from build123d import *

# Parameters (mm, degrees)
SKETCH2_R           = 45
BOSS_EXTRUDE3_DEPTH = 56
SKETCH4_W           = 90
SKETCH4_H           = 170
BOSS_EXTRUDE4_DEPTH = 30
SKETCH6_R           = 15
BOSS_EXTRUDE5_DEPTH = 170
SKETCH11_W          = 132.381260595
SKETCH11_H          = 110
CUT_EXTRUDE3_DEPTH  = 130


with BuildPart() as part:
    # Sketch2 → Boss-Extrude3 (new body)
    with BuildSketch(Plane.XY):
        Circle(SKETCH2_R)
        with BuildLine():
            Line((-4.5, 29.491665255), (4.5, 29.491665255))
            Line((4.5, 29.491665255), (4.5, 24.591665255))
            ThreePointArc((4.5, 24.591665255), (0, -25), (-4.5, 24.591665255))
            Line((-4.5, 24.591665255), (-4.5, 29.491665255))
        make_face(mode=Mode.SUBTRACT)
    extrude(amount=-BOSS_EXTRUDE3_DEPTH)

    # Sketch4 → Boss-Extrude4 (add)
    with BuildSketch(Plane(origin=(0, 0, -56), x_dir=(-1, 0, 0), z_dir=(0, 0, -1))):
        Rectangle(SKETCH4_W, SKETCH4_H)
    extrude(amount=BOSS_EXTRUDE4_DEPTH)

    # Sketch6 → Boss-Extrude5 (add)
    with BuildSketch(Plane(origin=(0, 85, 0), x_dir=(1, 0, 0), z_dir=(0, 1, 0))):
        with BuildLine():
            Line((45, 86), (38, 130))
            ThreePointArc((38, 130), (0, 168), (-38, 130))
            Line((-38, 130), (-45, 86))
            Line((-45, 86), (45, 86))
        make_face()
        with Locations(Location((0, 130, 0), (0, 0, 270))):
            Circle(SKETCH6_R, mode=Mode.SUBTRACT)
    extrude(amount=-BOSS_EXTRUDE5_DEPTH)

    # Sketch11 → Cut-Extrude3 (cut, symmetric)
    with BuildSketch(Plane(origin=(0, 0, 0), x_dir=(0, 0, -1), z_dir=(1, 0, 0))):
        with Locations((152.190630298, 0)):
            Rectangle(SKETCH11_W, SKETCH11_H)
    extrude(amount=CUT_EXTRUDE3_DEPTH, both=True, mode=Mode.SUBTRACT)


solid = part.part
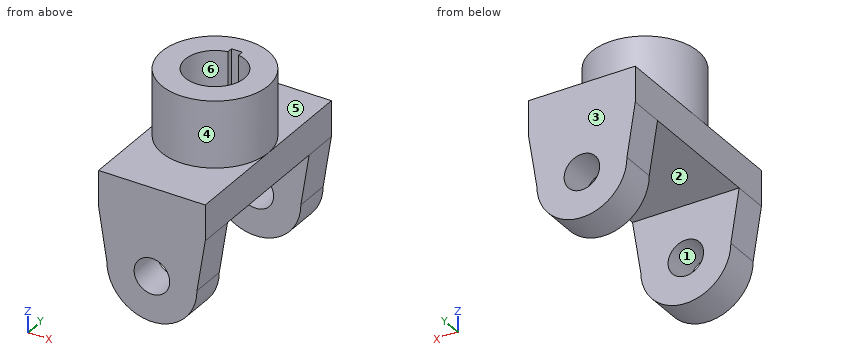
CAD build for the part. Positions are in the model's coordinates, mm. Face numbers are marked on the shaded views. A direction names the side the tool comes from. Round coordinates to 2 decimals unless told otherwise and drop trailing zeros. Order: outer loops, then holes, each group sorted by start corner. A loop starts at its lowest first (then second) coordinate and runs counter-clockwise, first axis right, second up. Notation, with made-up numbers: (48, 79) - (56, 79) arc R14 cw to (56, 106) - close; hole circle Ø4 at (20, 32.25). An arc over 180 degrees is marked (long way). Return JSON: item names as keys, results as strings.
(1) Cut at C-C (z = -157). Give the cut face in (x, y).
Answer key:
{"outline": "(-26.74, -85) - (26.74, -85) - (26.74, -55) - (-26.74, -55) - close; (-26.74, 55) - (26.74, 55) - (26.74, 85) - (-26.74, 85) - close"}
(2) Wall check: probe 1 along X at (y, z) = (1, -15); probe 2 along X at (y, z) = (-76.5, -130); probe 3 along Y at (x, z) = (0, -19.5). Give the ranges that are in metal, low to high. Write a range as from..to.
Answer key:
{"probe 1": "x = -44.99..-24.98, 24.98..44.99", "probe 2": "x = -38..-15, 15..38", "probe 3": "y = -45..-25, 29.49..45"}
(3) Tool access for the marked faces 1 and 2: list every direction of +Z, -Z, +X, -X, +Y, -Y with a clear straight run to the whole face (end or side of a thin tool).
Answer key:
{"face 1": "+Y, -Y", "face 2": "-Z, +X, -X"}
(4) Pin check, flat tips, straight feed: pin 1 Ø2 at (x, y) = (-29.5, -55) entering from +Z; pin 2 Ø5 at (x, y) = (16, -2.5) entering from -Z; pin 3 Ø24 at (x, z) = (0, -130) entering from -Y; pin 4 Ø2 at (y, z) = (66.5, -108.5) entering from +X. Stop position of each tip, or through.
Answer key:
{"pin 1": "stops at z = -56", "pin 2": "stops at z = -86", "pin 3": "passes through", "pin 4": "stops at x = 41.58"}
(5) Cut at A-A (x = 0). Give the cut face in (y, z), then the cut area to 3 significant figures.
Answer key:
{"outline": "(-85, -168) - (-55, -168) - (-55, -145) - (-85, -145) - close; (-85, -115) - (-55, -115) - (-55, -86) - (55, -86) - (55, -115) - (85, -115) - (85, -56) - (45, -56) - (45, 0) - (29.49, 0) - (29.49, -56) - (-25, -56) - (-25, 0) - (-45, 0) - (-45, -56) - (-85, -56) - close; (55, -168) - (85, -168) - (85, -145) - (55, -145) - close", "area": "10,200 mm^2"}
(6) Pull direction Y, two halves, no side cores. Call the marked faces 3, 4, 5 and 6: +Y half, -Y half, draft (parallel to the pull), parting line (faces both ways), or undercut.
Answer key:
{"face 3": "+Y half", "face 4": "parting line", "face 5": "draft", "face 6": "undercut"}
(7) Cut at B-B (y = -57.5). Give the cut face in (x, z), then the cut area to 3 significant figures.
Answer key:
{"outline": "(-45, -86) - (-38, -130) arc R38 ccw to (38, -130) - (45, -86) - (45, -56) - (-45, -56) - close; hole circle Ø30 at (0, -130)", "area": "7,910 mm^2"}
(8) Cut at D-D (z = -40.5). Give the cut face in (x, y), then the cut area to 3 significant figures.
Answer key:
{"outline": "circle Ø90 at (0, 0); hole (-4.5, 24.59) arc R25 ccw (long way) to (4.5, 24.59) - (4.5, 29.49) - (-4.5, 29.49) - close", "area": "4,360 mm^2"}
